```python
from build123d import *

# Parameters (mm, degrees)
SURFACE_EXTRUSION1_1_DEPTH = 30
EPAISSIR1_T1               = 2
EPAISSIR2_OUTLINE_W        = 50
EPAISSIR2_OUTLINE_H        = 20
EPAISSIR2_DEPTH            = 2
BOSS_EXTRU_1_DEPTH         = 54
CONG_1_R                   = 10


# Read off the part's stored shape, not the designer's step: Epaissir2
with BuildPart() as body_1:
    # Surface-Extrusion1: a surface, the sketch's curves swept straight by 30 mm
    with BuildLine(Plane(origin=(0, 0, 0), x_dir=(1, 0, 0), z_dir=(0, 1, 0)), mode=Mode.PRIVATE) as surface_extrusion1_1_path:
        Line((0, 0), (-50, 0))
        Line((-50, 0), (-50, 20))
        Line((-50, 20), (0, 20))
        Line((0, 20), (0, 0))
    surface_extrusion1_1 = Shell.extrude(surface_extrusion1_1_path.wire(), (0 * SURFACE_EXTRUSION1_1_DEPTH, 1 * SURFACE_EXTRUSION1_1_DEPTH, 0 * SURFACE_EXTRUSION1_1_DEPTH))
    add(Solid.thicken(surface_extrusion1_1, EPAISSIR1_T1))

    # Epaissir2 outline → Epaissir2 (add)
    with BuildSketch(Plane(origin=(0, 0, 0), x_dir=(1, 0, 0), z_dir=(0, 1, 0))):
        with Locations((-25, 10)):
            Rectangle(EPAISSIR2_OUTLINE_W, EPAISSIR2_OUTLINE_H)
    extrude(amount=EPAISSIR2_DEPTH)

    # Esquisse3 → Boss.-Extru.1 (add)
    with BuildSketch(Plane.ZY.offset(52)):
        Polygon((-22, 0), (-22, -9.980445305), (-20.597715591, -9.980445305), (-20.597715591, -3.819178115), (0.770065176, -3.819178115), (0.770065176, -9.980445305), (2, -9.980445305), (2, 0), align=None)
    extrude(amount=-BOSS_EXTRU_1_DEPTH)

    # Congé1
    # the kernel refuses this fillet: 10 mm, written as the material it adds along each edge
    with BuildSketch(Plane(origin=(-52, -3.819178115, 0.770065176), x_dir=(0, -1, 0), z_dir=(1, 0, 0))) as cong_1_piece_1:
        with BuildLine():
            CenterArc((10, 9.233857829), CONG_1_R, 180, 67.426190035)
            Line((0, 9.233857829), (-0.2, 9.233857829))
            Line((-0.2, 9.233857829), (-0.2, 0))
            Line((-0.2, 0), (0, -0.2))
            ThreePointArc((0, -0.2), (3.080633595, -0.2), (6.084492534, -0.184677157))
            Line((6.084492534, -0.184677157), (6.16126719, 0))
        make_face()
    extrude(amount=54)
    with BuildSketch(Plane(origin=(-52, -3.819178115, -20.597715591), x_dir=(0, 0, 1), z_dir=(1, 0, 0))) as cong_1_piece_2:
        with BuildLine():
            CenterArc((9.233857829, 10), CONG_1_R, 202.573809965, 67.426190035)
            Line((0, 6.16126719), (-0.184677157, 6.084492534))
            ThreePointArc((-0.184677157, 6.084492534), (-0.2, 3.080633595), (-0.2, 0))
            Line((-0.2, 0), (0, -0.2))
            Line((0, -0.2), (9.233857829, -0.2))
            Line((9.233857829, -0.2), (9.233857829, 0))
        make_face()
    extrude(amount=54)


solid = body_1.part
```
Read the model definition and answer for the solid it produces. Units are mm, in the model's axes. A direction names the side the tool comes from. Coordinates: 2 decimals unless noted, no trailing zeros. Write each loop counter-clockwise with the first axis right and the second up, starting at its lowest first coordinate (ties: lowest second). Pieces come first, ordered by that corner, then holes. Notation, with made-up numbers: (-19, 82.25) - (25, 82.25) arc R16 cw to (25, 108.25) - close; hole circle Ø6 at (13.5, 87.25). An arc over 180 degrees is marked (long way). Answer as a JSON object with one key per item and string values. Group by question number.
1. A cutting plane is placed at D-D (z = -4.25). Determine the outline of the cut face in (x, y), plus the area to 3 significant figures.
2. The mould has two halves that part along Z. Classify faces 4 (the flat face through (-25, 16, 0)), 5 (the flat face through (2, 10, -10)), 6 (the flat face through (-25, 10, 2)): +Z half, -Z half, draft (parallel to the pull), parting line (faces both ways), or undercut.
3. Consider L1, parallel to Z at x = -23, y = 8; L2, parallel to X at y = 13.5, z = -16.5; L3, parallel to Y at x = -42, z = -8.5. Determine where each line is inside the solid, lowest interval first. Write a range as [from, to].
4. Which of the six approach directions +Z, -Z, +X, -X, +Y, -Y give full straight-line access (tool end or side, diameter ignored) to faces 1 (the flat face through (-25, -3.819, -10)), 2 (the flat face through (-52, 10, -10)), 3 (the flat face through (0, 16, -10))?
5. A cutting plane is placed at A-A (y = 18.5). Determine the outline of the cut face in (x, z), plus the area to 3 significant figures.
6. A cutting plane is placed at C-C (z = -14.75). Determine the outline of the cut face in (x, y).
7. A cutting plane is placed at B-B (x = -7). Determine the outline of the cut face in (y, z), plus the area to 3 significant figures.
8. Each of these flat-tipped pins is pushed along its axis until it touches: P1, Ø10, axis at x = -46.5, z = -10, coming from the +Y side; P2, Ø2.5, axis at x = -12, z = -10.5, coming from the -Y side; P3, Ø1.5, axis at x = -12.5, z = -7.5, coming from the +Y side; P4, Ø2, axis at x = -5, z = -18, coming from the -Y side. Where does it stop, or does it pass through?
Worked out:
{
 "1": {"outline": "(-52, -4.75) - (2, -4.75) - (2, 30) - (0, 30) - (0, 2) - (-50, 2) - (-50, 30) - (-52, 30) - close", "area": "477 mm²"},
 "2": {"face 4": "undercut", "face 5": "draft", "face 6": "+Z half"},
 "3": {"L1": "z = [-22, -20], [0, 2]", "L2": "x = [-52, -50], [0, 2]", "L3": "y = [-3.82, 2]"},
 "4": {"face 1": "+X, -X, -Y", "face 2": "+Z, -Z, -X, +Y, -Y", "face 3": "+Y"},
 "5": {"outline": "(-52, -22) - (2, -22) - (2, 2) - (-52, 2) - close; hole (-50, -20) - (0, -20) - (0, 0) - (-50, 0) - close", "area": "296 mm²"},
 "6": {"outline": "(-52, -4.41) - (2, -4.41) - (2, 30) - (0, 30) - (0, 2) - (-50, 2) - (-50, 30) - (-52, 30) - close"},
 "7": {"outline": "(-9.98, -22) - (30, -22) - (30, -20) - (2, -20) - (2, 0) - (30, 0) - (30, 2) - (-9.98, 2) - (-9.98, 0.77) arc R10 cw to (-3.82, -8.46) - (-3.82, -11.36) arc R10 cw to (-9.98, -20.6) - close", "area": "299 mm²"},
 "8": {"P1": "stops at y = 30", "P2": "stops at y = -3.83", "P3": "stops at y = 2", "P4": "stops at y = -7.36"}
}
